from build123d import *

# Parameters (mm, degrees)
SKETCH1_W                                    = 46
SKETCH1_H                                    = 46
BOSS_EXTRUDE1_DEPTH                          = 65
SKETCH3_W                                    = 75
SKETCH3_H                                    = 75
SKETCH3_W_2                                  = 52
SKETCH3_H_2                                  = 52
SKETCH3_W_3                                  = 23
SKETCH3_H_3                                  = 46
BOSS_EXTRUDE2_DEPTH                          = 5
SKETCH8_W                                    = 75
SKETCH8_H                                    = 75
SKETCH8_W_2                                  = 52
SKETCH8_H_2                                  = 52
BOSS_EXTRUDE3_DEPTH                          = 5.047079132
FILLET1_R                                    = 2
CBORE_FOR_M6_HEX_SOCKET_HEAD_CAP_SCR_2_COUNT = 2
CBORE_FOR_M6_HEX_SOCKET_HEAD_CAP_SCR_2_PITCH = 50
CBORE_FOR_M6_HEX_SOCKET_HEAD_CAP_SCR_3_COUNT = 2
CBORE_FOR_M6_HEX_SOCKET_HEAD_CAP_SCR_3_PITCH = 63.5
CBORE_FOR_M6_HEX_SOCKET_HEAD_CAP_SCR_4_COUNT = 2
CBORE_FOR_M6_HEX_SOCKET_HEAD_CAP_SCR_4_PITCH = 80.822336022
CHAMFER2_SIZE                                = 2
FILLET2_R                                    = 1.2


with BuildPart() as part:
    # Sketch1 → Boss-Extrude1 (new body)
    with BuildSketch(Plane(origin=(0, 0, 0), x_dir=(0, 1, 0), z_dir=(0, 0, 1))):
        Polygon((-26.156583063, 30.146094376), (-29.048003873, 30.146094376), (-29.048003873, -21.853905624), (22.951996127, -21.853905624), (22.951996127, 30.146094376), (15.339697873, 30.146094376), align=None)
        with Locations((-3.048003873, 4.146094376)):
            Rectangle(SKETCH1_W, SKETCH1_H, mode=Mode.SUBTRACT)
    extrude(amount=BOSS_EXTRUDE1_DEPTH)

    # Sketch3 → Boss-Extrude2 (add)
    # profile 1 of 5: a face of its own
    with BuildSketch(Plane(origin=(0, 0, 0), x_dir=(1, 0, 0), z_dir=(0, 0, -1))):
        with Locations((-4.146094376, 3.048003873)):
            Rectangle(SKETCH3_W, SKETCH3_H)
        with Locations((-4.146094376, 3.048003873)):
            Rectangle(SKETCH3_W_2, SKETCH3_H_2, mode=Mode.SUBTRACT)
    # profile 2 of 5: a face of its own
    with BuildSketch(Plane(origin=(0, 0, 0), x_dir=(1, 0, 0), z_dir=(0, 0, -1))):
        Polygon((21.853905624, 29.048003873), (-4.146094376, 29.048003873), (-4.146094376, 26.048003873), (18.853905624, 26.048003873), (18.853905624, -19.951996127), (-4.146094376, -19.951996127), (-4.146094376, -22.951996127), (21.853905624, -22.951996127), align=None)
    # profile 3 of 5: a face of its own
    with BuildSketch(Plane(origin=(0, 0, 0), x_dir=(1, 0, 0), z_dir=(0, 0, -1))):
        Polygon((-4.146094376, 26.048003873), (-4.146094376, 29.048003873), (-30.146094376, 29.048003873), (-30.146094376, -22.951996127), (-4.146094376, -22.951996127), (-4.146094376, -19.951996127), (-27.146094376, -19.951996127), (-27.146094376, 26.048003873), align=None)
    # profile 4 of 5: a face of its own
    with BuildSketch(Plane(origin=(0, 0, 0), x_dir=(1, 0, 0), z_dir=(0, 0, -1))):
        with Locations((7.353905624, 3.048003873)):
            Rectangle(SKETCH3_W_3, SKETCH3_H_3)
    # profile 5 of 5: a face of its own
    with BuildSketch(Plane(origin=(0, 0, 0), x_dir=(1, 0, 0), z_dir=(0, 0, -1))):
        with Locations((-15.646094376, 3.048003873)):
            Rectangle(SKETCH3_W_3, SKETCH3_H_3)
    extrude(amount=BOSS_EXTRUDE2_DEPTH)

    # Sketch8 → Boss-Extrude3 (add)
    with BuildSketch(Plane.XY):
        with Locations((-4.146094376, -3.048003873)):
            Rectangle(SKETCH8_W, SKETCH8_H)
        with Locations((-4.146094376, -3.048003873)):
            Rectangle(SKETCH8_W_2, SKETCH8_H_2, mode=Mode.SUBTRACT)
    extrude(amount=BOSS_EXTRUDE3_DEPTH)

    # Fillet1
    fillet1_edges = [part.edges().sort_by_distance(p)[0] for p in [
        (21.853905624, 22.951996127, 35.023539566),
        (21.853905624, -29.048003873, 35.023539566),
        (-30.146094376, -29.048003873, 35.023539566),
        (-30.146094376, 22.951996127, 35.023539566),
        (-41.646094376, -40.548003873, 0.023539566),
        (33.353905624, -40.548003873, 0.023539566),
        (33.353905624, 34.451996127, 0.023539566),
        (-41.646094376, 34.451996127, 0.023539566),
    ]]
    fillet(fillet1_edges, radius=FILLET1_R)

    # Sketch15 → CBORE for M6 Hex Socket Head Cap Screw2 (revolve, cut)
    with BuildSketch(Plane(origin=(-35.896094376, 21.951996127, 5.047079132), x_dir=(0, -1, 0), z_dir=(1, 0, 0))):
        Polygon((0, 0), (0, 10.047079132), (3.3, 10.047079132), (3.3, 6.4), (5.5, 6.4), (5.5, 0.025), (5.525, 0), align=None)
    cbore_for_m6_hex_socket_head_cap_screw2 = revolve(axis=Axis((-35.896094376, 21.951996127, 11.397079132), (0, 0, -1)), mode=Mode.SUBTRACT)

    # CBORE for M6 Hex Socket Head Cap Scr 2: CBORE for M6 Hex Socket Head Cap Screw2 ×2
    with Locations(*[(0, -i * CBORE_FOR_M6_HEX_SOCKET_HEAD_CAP_SCR_2_PITCH, 0) for i in range(1, CBORE_FOR_M6_HEX_SOCKET_HEAD_CAP_SCR_2_COUNT)]):
        add(cbore_for_m6_hex_socket_head_cap_screw2, mode=Mode.SUBTRACT)

    # CBORE for M6 Hex Socket Head Cap Scr 3: CBORE for M6 Hex Socket Head Cap Screw2 ×2
    with Locations(*[(i * CBORE_FOR_M6_HEX_SOCKET_HEAD_CAP_SCR_3_PITCH, 0, 0) for i in range(1, CBORE_FOR_M6_HEX_SOCKET_HEAD_CAP_SCR_3_COUNT)]):
        add(cbore_for_m6_hex_socket_head_cap_screw2, mode=Mode.SUBTRACT)

    # CBORE for M6 Hex Socket Head Cap Scr 4: CBORE for M6 Hex Socket Head Cap Screw2 ×2
    with Locations(*[Vector(0.7856739006278309, -0.6186408666360874, 0) * (i * CBORE_FOR_M6_HEX_SOCKET_HEAD_CAP_SCR_4_PITCH) for i in range(1, CBORE_FOR_M6_HEX_SOCKET_HEAD_CAP_SCR_4_COUNT)]):
        add(cbore_for_m6_hex_socket_head_cap_screw2, mode=Mode.SUBTRACT)

    # Chamfer2
    chamfer2_edges = [part.edges().sort_by_distance(p)[0] for p in [
        (33.353905624, -3.048003873, -5),
        (-4.146094376, 34.451996127, -5),
        (-4.146094376, -40.548003873, -5),
        (-41.646094376, -3.048003873, -5),
        (32.768119187, -39.962217436, -5),
        (-41.060307938, -39.962217436, -5),
        (-41.060307938, 33.866209689, -5),
        (32.768119187, 33.866209689, -5),
    ]]
    chamfer(chamfer2_edges, length=CHAMFER2_SIZE)

    # Fillet2
    fillet2_edges = [part.edges().sort_by_distance(p)[0] for p in [
        (18.853905624, -26.048003873, 32.5),
        (18.853905624, 19.951996127, 32.5),
        (-27.146094376, 19.951996127, 32.5),
        (-27.146094376, -26.048003873, 32.5),
    ]]
    fillet(fillet2_edges, radius=FILLET2_R)


solid = part.part
Verification items for the finished model (mm, model axes). A direction names the side the tool comes from. Coordinates: 2 decimals unless noted, no trailing zeros. Order: outer loops, then holes, each group sorted by start corner. A loop starts at its lowest first (then second) coordinate and runs counter-clockwise, first axis right, second up. Notation, with made-up numbers: M 44.25,6 L 85.25,6 A14 ccw 85.25,21 Z; hole C 72.5,-30.75 d5. An arc over 180 degrees is marked long. Write each question's results on one line, items separated by ' | '.
1) Gauge pin test, flat ends, axial feed: pin 1 Ø1.5 at (x, z) = (-26.5, 21) entering from +Y; pin 2 Ø2 at (x, y) = (-14.5, 15.5) entering from +Z; pin 3 Ø2 at (y, z) = (11.5, 35.5) entering from +X. Record the tip position at first contact, or that the pin passes through.
Solved:
pin 1: stops at y = 22.95 | pin 2: stops at z = 0 | pin 3: stops at x = 21.85
2) Access from +Z, -Z, +X, -X, +Y, -Y to the whole of each face (thin tool, end or side, straight path). Record for faces 4 (the face through (-32.675, 22.667, -3.151)), 5 (the face through (28, 26, -1.353)), 6 (the face through (-29.576, -28.447, 35.443)).
Solved:
face 4: +Z, -Z | face 5: +Z | face 6: +Z, -X, -Y
3) Section check B-B on y = -10. Record the cut outline in (x, z), plus the area to 3 significant figures.
Solved:
outline: M -41.65,-3 L -39.65,-5 L 31.35,-5 L 33.35,-3 L 33.35,5.05 L 21.85,5.05 L 21.85,65 L 18.85,65 L 18.85,0 L -27.15,0 L -27.15,65 L -30.15,65 L -30.15,5.05 L -41.65,5.05 Z | area: 877 mm²
4) Section check A-A on z = 57. Record the cut outline in (x, y).
Solved:
outline: M -30.15,-27.05 A2 ccw -28.15,-29.05 L 19.85,-29.05 A2 ccw 21.85,-27.05 L 21.85,20.95 A2 ccw 19.85,22.95 L -28.15,22.95 A2 ccw -30.15,20.95 Z; hole M -27.15,-24.85 A1.2 ccw -25.95,-26.05 L 17.65,-26.05 A1.2 ccw 18.85,-24.85 L 18.85,18.75 A1.2 ccw 17.65,19.95 L -25.95,19.95 A1.2 ccw -27.15,18.75 Z
5) Section check C-C on x = 7.5. Record the cut outline in (y, z), plus the area to 3 significant figures.
Solved:
outline: M -40.55,-3 L -38.55,-5 L 32.45,-5 L 34.45,-3 L 34.45,5.05 L 22.95,5.05 L 22.95,65 L 19.95,65 L 19.95,0 L -26.05,0 L -26.05,65 L -29.05,65 L -29.05,5.05 L -40.55,5.05 Z | area: 877 mm²
6) Release check for a two-part mould opening along X. For faces 1 (the face through (-27.4, -7, 65)), 2 (the face through (-30.527, -26.856, 1.879)), 3 (the face through (21.854, -3, 35)) record: pulls with the +X half, pulls with the -X half, needs draft (parallel to the pull), parting line crosses it, or undercut.
Solved:
face 1: needs draft | face 2: undercut | face 3: pulls with the +X half
7) Scan lines: line 1 along Y through (x, z) = (-17.5, 61); line 2 along X through (y, z) = (-4, 45); line 3 along Y through (x, z) = (-23, 3.5). Record each from-to range of solid material in increasing order. Write a range as [from, to].
Solved:
line 1: y = [-29.05, -26.05], [19.95, 22.95] | line 2: x = [-30.15, -27.15], [18.85, 21.85] | line 3: y = [-40.55, -26.05], [19.95, 34.45]
